Autodesk Fusion 360 part; units mm, degrees
sketch "Sketch1" plane through (0, 0, 0) normal (0, 1, 0) x (1, 0, 0)
  circle A0 centre (0, 40) radius 1.4
  circle A1 centre (-25, 0) radius 1.4
  circle A2 centre (25, 0) radius 1.4
  line L0 (-25, 0) -> (25, 0) construction
  line L1 (0, 0) -> (0, 40) construction
  line L2 (-27.3744, 1.484) -> (-2.3744, 41.484)
  line L3 (25, -2.8) -> (-25, -2.8)
  line L4 (27.3744, 1.484) -> (2.3744, 41.484)
  arc A3 (25, -2.8) -> (27.3744, 1.484) centre (25, 0) ccw
  arc A4 (-27.3744, 1.484) -> (-25, -2.8) centre (-25, 0) ccw
  arc A5 (2.3744, 41.484) -> (-2.3744, 41.484) centre (0, 40) ccw
  circle A6 centre (-10, 20) radius 2.05
  circle A7 centre (10, 20) radius 2.05
  circle A8 centre (0, 0) radius 2.05
  line L5 (0, 0) -> (0, -2.8) construction
  circle A9 centre (0, 12.5) radius 3.5
  line L6 (0, 12.5) -> (-10, 20) construction
  line L7 (0, 12.5) -> (0, 0) construction
  dimension "d16" = 2.8
  dimension "d19" = 50
  dimension "d21" = 40
  dimension "d22" = 1.4
  dimension "d23" = 1.4
  dimension "d24" = 4.1
  dimension "d28" = 7
  dimension "d36" = 20
  dimension "d37" = 10
extrude "Extrude1" add sketch "Sketch1" along normal blind 4 contours L2 L3 L4 A3 A4 A5 | A9 makes body 1
extrude "Extrude2" add sketch "Sketch1" along normal blind 7.5 separate body contours A0 | A1 | A2 | L2 L3 L4 A3 A4 A5 makes body 2
extrude "Extrude3" add sketch "Sketch1" along normal blind 1 contours A0 | A1 | A2 bodies 1
extrude "Extrude5" add sketch "Sketch1" along normal blind 1 contours A6 | A7 | A8 bodies 2
extrude "Extrude6" add sketch "Sketch1" along normal blind 5 separate body contours L2 L3 L4 A3 A4 A5 | A6 | A7 | A8 | A9 makes body 3
hidden bodies 2 3
equation "holeDiam = 2.8 mm"
equation "RodHoleDiam = 4.1 mm"
equation "d16 = holeDiam"
equation "d22 = holeDiam / 2"
equation "d23 = holeDiam / 2"
equation "d24 = RodHoleDiam"
Work out the finished part from the listing and answer in its coordinate system (mm). A direction names the side the tool comes from. Coordinates: 2 decimals unless noted, no trailing zeros. Write each loop counter-clockwise with the first axis right and the second up, starting at its lowest first coordinate (ties: lowest second). Pieces come first, ordered by that corner, then holes. Notation, with made-up numbers: (89.5, -25) - (116.5, -25) arc R26 ccw to (116.5, 4) - close; hole circle Ø10 at (31, -23.75). An arc over 180 degrees is marked (long way). Answer as a JSON object with one key per item and string values.
Q1. For a pull along Z with two mould halves and no side action, classify faces 1 (the cylindrical face through (-27.43, 1.97, 1.39)), 2 (the cylindrical face through (-0.267, 1.972, 2.033)), 3 (the flat face through (0, 4, -15)), 4 (the cylindrical face through (26.29, 2.48, -0.54)) as pulls with the +Z half, pulls with the -Z half, needs draft (parallel to the pull), parting line crosses it, or undercut.
Results list:
{"face 1": "parting line crosses it", "face 2": "undercut", "face 3": "needs draft", "face 4": "undercut"}
Q2. Find section D-D (z = -20). Write down the section's boundary in (x, y), plus the area to 3 significant figures.
Results list:
{"outline": "(-15.8, 0) - (-12.05, 0) - (-12.05, 4) - (-15.8, 4) - close; (-7.95, 0) - (7.95, 0) - (7.95, 4) - (-7.95, 4) - close; (12.05, 0) - (15.8, 0) - (15.8, 4) - (12.05, 4) - close", "area": "93.6 mm^2"}
Q3. Which of the six approach directions +Z, -Z, +X, -X, +Y, -Y give full straight-line access (tool end or side, diameter ignored) to faces 5 (the cylindrical face through (8.5, 2, -18.6)), 6 (the cylindrical face through (-23.71, 2.48, -0.54))?
Results list:
{"face 5": "+Y, -Y", "face 6": "+Y"}
Q4. Find section B-B (z = 0). Write down the section's boundary in (x, y).
Results list:
{"outline": "(-27.8, 0) - (-2.05, 0) - (-2.05, 4) - (-23.6, 4) - (-23.6, 1) - (-26.4, 1) - (-26.4, 4) - (-27.8, 4) - close; (2.05, 0) - (27.8, 0) - (27.8, 4) - (26.4, 4) - (26.4, 1) - (23.6, 1) - (23.6, 4) - (2.05, 4) - close"}
Q5. Find section C-C (y = 2.65). Write down the section's boundary in (x, z), plus the area to 3 significant figures.
Results list:
{"outline": "(-27.37, -1.48) - (-2.37, -41.48) arc R2.8 ccw to (2.37, -41.48) - (27.37, -1.48) arc R2.8 ccw to (25, 2.8) - (-25, 2.8) arc R2.8 ccw to start; hole circle Ø2.8 at (-25, 0); hole circle Ø4.1 at (-10, -20); hole circle Ø4.1 at (0, 0); hole circle Ø2.8 at (0, -40); hole circle Ø4.1 at (10, -20); hole circle Ø2.8 at (25, 0)", "area": "1,370 mm^2"}
Q6. Given pin 1 Ø1.4 at (x, z) = (0, -40) entering from +Y; pin 2 Ø1 at (y, z) = (3.5, -31.5) entering from +X, each flat-ended and moving along its own axis, determine where each tip first touches the part or whether it passes through.
Results list:
{"pin 1": "stops at y = 1", "pin 2": "stops at x = 8.93"}
Q7. Find section A-A (x = 0). Write down the section's boundary in (y, z).
Results list:
{"outline": "(0, -42.8) - (4, -42.8) - (4, -41.4) - (1, -41.4) - (1, -38.6) - (4, -38.6) - (4, -2.05) - (0, -2.05) - close; (0, 2.05) - (4, 2.05) - (4, 2.8) - (0, 2.8) - close"}
Q8. Consider L1, parallel to Z at x = 0, y = 2.3; L2, parallel to X at y = 2.4, z = 0; L3, parallel to X at y = 0.4, z = -20. Determine where each line is inside the solid, lowest interval first. Write a range as from..to.
Results list:
{"L1": "z = -42.8..-41.4, -38.6..-2.05, 2.05..2.8", "L2": "x = -27.8..-26.4, -23.6..-2.05, 2.05..23.6, 26.4..27.8", "L3": "x = -15.8..-12.05, -7.95..7.95, 12.05..15.8"}
